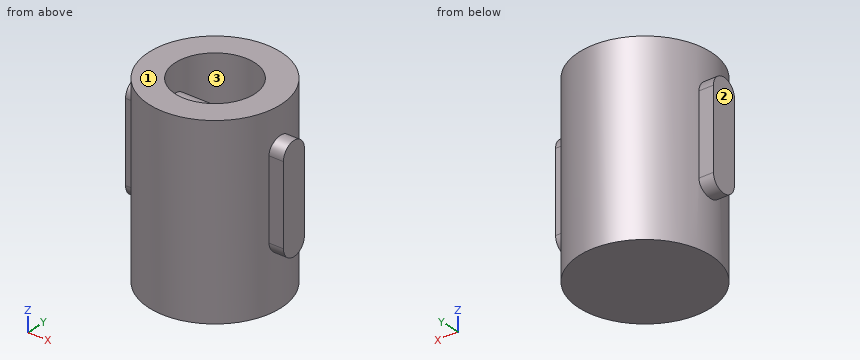
from build123d import *

# Parameters (mm, degrees)
F0_R     = 25
F1_DEPTH = 70
F3_D     = 30
F3_DEPTH = 50
F3_TIP   = 9.0129092854
F4_W     = 10
F4_H     = 30
F5_DEPTH = 30


with BuildPart() as f1:
    # F0 (on Top) → F1 (new body)
    with BuildSketch(Plane.XY):
        Circle(F0_R)
    extrude(amount=F1_DEPTH)

    # F3
    with Locations(Plane.XY.offset(70)):
        with Locations((0, 0)):
            Hole(F3_D / 2, depth=F3_DEPTH)
            with Locations((0, 0, -(F3_DEPTH + F3_TIP / 2))):  # 118° drill point
                Cone(0, F3_D / 2, F3_TIP, mode=Mode.SUBTRACT)

    # F4 (on Right) → F5 (join, symmetric)
    with BuildSketch(Plane.YZ):
        with BuildLine():
            ThreePointArc((5, 54.499398917), (0, 59.499398917), (-5, 54.499398917))
            Line((-5, 54.499398917), (5, 54.499398917))
        make_face()
        with Locations((0, 39.499398917)):
            Rectangle(F4_W, F4_H)
        with BuildLine():
            Line((5, 24.499398917), (-5, 24.499398917))
            ThreePointArc((-5, 24.499398917), (0, 19.499398917), (5, 24.499398917))
        make_face()
    extrude(amount=F5_DEPTH, both=True)


solid = f1.part
Part model, mm, in its own coordinate system. Face numbers are marked on the shaded views. Round coordinates to 2 decimals unless told otherwise and drop trailing zeros. Loops run counter-clockwise (first coordinate to the right, second up) from the corner with the lowest first, then second, coordinate; pieces in that order, holes last. Notation, with made-up numbers: (62, 32) - (103, 32) arc R20 cw to (103, 54) - close; hole circle Ø11 at (-9.75, 19). An arc over 180 degrees is marked (long way). Answer as a JSON object with one key per item and string values.
Item 1: Wall check: L1, parallel to Y at x = 0, z = 33; L2, parallel to Y at x = 0, z = 57; L3, parallel to Z at x = 12, y = 3.5. Give the ranges that are in metal, low to high.
Output:
{"L1": "-25 to -15, -5 to 5, 15 to 25", "L2": "-25 to -15, -4.33 to 4.33, 15 to 25", "L3": "0 to 18.5, 20.93 to 58.07"}
Item 2: Pin check, flat tips, straight feed: pin 1 (22.5 mm diameter, centred on x = 3.5, z = 43.5, fed in from -Y); pin 2 (2 mm diameter, centred on x = -0.5, z = 29, fed in from +Y); pin 3 (12 mm diameter, centred on x = -13, y = -5, fed in from -Z); pin 4 (12 mm diameter, centred on y = 13.5, z = 10.5, fed in from -X). Stop position of each tip, or through.
Output:
{"pin 1": "y = -25", "pin 2": "y = 25", "pin 3": "z = 0", "pin 4": "x = -23.85"}
Item 3: Band-saw the part on A-A on z = 50.5. List the corners of the cut face in (x, y), plus the area to 3 significant figures.
Output:
{"outline": "(-30, -5) - (-24.49, -5) arc R25 ccw to (24.49, -5) - (30, -5) - (30, 5) - (24.49, 5) arc R25 ccw to (-24.49, 5) - (-30, 5) - close; hole (-14.14, -5) arc R15 ccw to (14.14, -5) - close; hole (-14.14, 5) - (14.14, 5) arc R15 ccw to start", "area": "1,650 mm2"}
Item 4: Pull direction X, two halves, no side cores. Call the marked faces 1, 2 and 3: pulls with the +X half, pulls with the -X half, needs draft (parallel to the pull), parting line crosses it, or undercut.
Output:
{"face 1": "needs draft", "face 2": "pulls with the -X half", "face 3": "undercut"}
Item 5: Band-saw the part on B-B on y = -20.5. List the corners of the cut face in (x, z).
Output:
{"outline": "(-14.31, 0) - (14.31, 0) - (14.31, 70) - (-14.31, 70) - close"}
Item 6: Band-saw the part on C-C on y = 16. List the corners of the cut face in (x, z), plus the area to 3 significant figures.
Output:
{"outline": "(-19.21, 0) - (19.21, 0) - (19.21, 70) - (-19.21, 70) - close", "area": "2,690 mm2"}
